Work out the finished part from the listing and answer in its coordinate system (mm). Give positions to 0.01 mm unless a question says otherwise; leave off trailing zeros. Order: outer loops, then holes, each group sorted by start corner. A loop starts at its lowest first (then second) coordinate and runs counter-clockwise, first axis right, second up. Notation, with made-up numbers: (-22, -30.75) - (-15, -30.75) arc R23 ccw to (-15, -19.75) - close; hole circle Ø3 at (48, 39). An arc over 180 degrees is marked (long way). Write each question's results on one line, items separated by ' | '.
from build123d import *

# Parameters (mm, degrees)
SKETCH1_R           = 17
SKETCH1_R_2         = 13
BOSS_EXTRUDE1_DEPTH = 4
SKETCH2_R           = 1.6
SKETCH2_R_2         = 1.5
CUT_EXTRUDE1_DEPTH  = 248.51565607


with BuildPart() as part:
    # Sketch1 → Boss-Extrude1 (new, symmetric)
    with BuildSketch(Plane(origin=(0, 0, 0), x_dir=(0, 0, -1), z_dir=(1, 0, 0))):
        with BuildLine():
            Line((-219.069767442, 24.666515623), (-9.76744186, 59.199637495))
            ThreePointArc((-9.76744186, 59.199637495), (60, 0), (-9.76744186, -59.199637495))
            Line((-9.76744186, -59.199637495), (-219.069767442, -24.666515623))
            ThreePointArc((-219.069767442, -24.666515623), (-240, 0), (-219.069767442, 24.666515623))
        make_face()
        Circle(SKETCH1_R, mode=Mode.SUBTRACT)
        with Locations((-215, 0)):
            Circle(SKETCH1_R_2, mode=Mode.SUBTRACT)
    extrude(amount=BOSS_EXTRUDE1_DEPTH, both=True)

    # Sketch2 → Cut-Extrude1 (cut, through all)
    with BuildSketch(Plane(origin=(4, 0, 0), x_dir=(0, 0, -1), z_dir=(1, 0, 0))):
        with Locations((0, 20)):
            Circle(SKETCH2_R)
        with Locations((20, 0)):
            Circle(SKETCH2_R)
        with Locations((0, -20)):
            Circle(SKETCH2_R)
        with Locations((-20, 0)):
            Circle(SKETCH2_R)
        with Locations((-215, 15)):
            Circle(SKETCH2_R_2)
        with Locations((-200, 0)):
            Circle(SKETCH2_R_2)
        with Locations((-215, -15)):
            Circle(SKETCH2_R_2)
        with Locations((-230, 0)):
            Circle(SKETCH2_R_2)
    extrude(amount=-CUT_EXTRUDE1_DEPTH, mode=Mode.SUBTRACT)


solid = part.part
1. A cutting plane is placed at D-D, the plane y = 39. Write down the section's boundary in (x, z), then the cut area to 3 significant figures.
Answer list:
outline: (-4, -45.6) - (4, -45.6) - (4, 132.2) - (-4, 132.2) - close | area: 1,420 mm^2
2. A cutting plane is placed at B-B, the plane y = -7. Write down the section's boundary in (x, z).
Answer list:
outline: (-4, -59.59) - (4, -59.59) - (4, -15.49) - (-4, -15.49) - close; (-4, 15.49) - (4, 15.49) - (4, 204.05) - (-4, 204.05) - close; (-4, 225.95) - (4, 225.95) - (4, 239) - (-4, 239) - close
3. A cutting plane is placed at A-A, the plane x = 1.5. State how many separate pieces and enclosed holes the cut face has, then the cut area to 3 significant figures.
Answer list:
separate pieces: 1 | enclosed holes: 10 | area: 23,700 mm^2
4. Straight lines are drawn through the part: line 1 (Y direction, x = -0.75, z = 0); line 2 (Z direction, x = 2.5, y = -3); line 3 (Z direction, x = 1.75, y = 8). For each, find the intervals that lie inside material, in ascending order. Write a range as [from, to].
Answer list:
line 1: [-60, -21.6], [-18.4, -17], [17, 18.4], [21.6, 60] | line 2: [-59.92, -16.73], [16.73, 202.35], [227.65, 239.82] | line 3: [-59.46, -15], [15, 204.75], [225.25, 238.69]
5. Given P1, Ø2.5, axis at y = 20, z = 0, coming from the +X side; P2, Ø4, axis at x = -0.5, y = 44, coming from the -Z side; P3, Ø1, axis at x = -3, y = 17.5, coming from the -Z side, each flat-ended and moving along its own axis, determine where each tip first touches the part or whether it passes through.
Answer list:
P1: through | P2: z = -42.85 | P3: z = -57.54
6. Determine the mould class of faces 1 (the face through (-0.056, 0.572, 227.987)), 2 (the face through (0.06, 41.69, 115.88)), 3 (the face through (-4, 1, 55)), 4 (the face through (-0.056, 14.334, -9.139)) for opening direction Z: +Z half, -Z half, draft (parallel to the pull), parting line (faces both ways), or undercut.
Answer list:
face 1: undercut | face 2: +Z half | face 3: draft | face 4: undercut
7. A cutting plane is placed at C-C, the plane z = 144. Write down the section's boundary in (x, y).
Answer list:
outline: (-4, -37.05) - (4, -37.05) - (4, 37.05) - (-4, 37.05) - close
